```python
from build123d import *

# Parameters (mm, degrees)
SKETCH1_R           = 101.6
BOSS_EXTRUDE1_DEPTH = 457.2
SKETCH2_W           = 3.175
SKETCH2_H           = 88.9
BOSS_EXTRUDE3_DEPTH = 139.7
SKETCH2_3_W         = 88.9
SKETCH2_3_H         = 88.9
BOSS_EXTRUDE4_DEPTH = 3.175


with BuildPart() as part:
    # Sketch1 → Boss-Extrude1 (new body)
    with BuildSketch(Plane(origin=(0, 0, 0), x_dir=(1, 0, 0), z_dir=(0, 1, 0))):
        Circle(SKETCH1_R)
    extrude(amount=BOSS_EXTRUDE1_DEPTH)

    # Sketch2 → Boss-Extrude3 (add)
    with BuildSketch(Plane(origin=(0, 457.2, 0), x_dir=(1, 0, 0), z_dir=(0, 1, 0))):
        with Locations((46.0375, 0)):
            Rectangle(SKETCH2_W, SKETCH2_H)
        with Locations((-46.0375, 0)):
            Rectangle(SKETCH2_W, SKETCH2_H)
    extrude(amount=BOSS_EXTRUDE3_DEPTH)

    # Sketch2<3> → Boss-Extrude4 (add)
    with BuildSketch(Plane(origin=(0, 457.2, 0), x_dir=(1, 0, 0), z_dir=(0, 1, 0))):
        Rectangle(SKETCH2_3_W, SKETCH2_3_H)
    extrude(amount=BOSS_EXTRUDE4_DEPTH)


solid = part.part
```
Model file for the job. Use its own axes, mm. A direction names the side the tool comes from. Coordinates: 2 decimals unless noted, no trailing zeros. Order: outer loops, then holes, each group sorted by start corner. A loop starts at its lowest first (then second) coordinate and runs counter-clockwise, first axis right, second up. Notation, with made-up numbers: (-20, 60) -> (-8, 60) arc R23 cw to (-8, 89) -> close; hole circle Ø9 at (57.5, 80). An arc over 180 degrees is marked (long way). Answer as a JSON object with one key per item and string values. Group by question number.
1) Cut at D-D, the plane y = 219. Write the cut outline in (x, z).
2) Pull direction X, two halves, no side cores. Call faces 1 (the face through (-1, 457.2, -47)), 2 (the face through (-47.625, 526, 1)), 3 (the face through (-1, 460.375, -1)): +X half, -X half, draft (parallel to the pull), parting line (faces both ways), or undercut.
3) Cut at B-B, the plane x = 0. Write the cut outline in (y, z) (3 decimals).
4) Cut at A-A, the plane y = 469.5. Write the cut outline in (x, z) (3 decimals), then the cut area to 3 significant figures.
5) Cut at C-C, the plane z = 0. Write the cut outline in (x, y) (3 decimals), then the cut area to 3 significant figures.
6) Flat gauge pins, fed straight in: pin 1 (1.5 mm diameter, centred on y = 426, z = 6.5, fed in from +X); pin 2 (6 mm diameter, centred on x = 50, z = 51.5, fed in from +Y); pin 3 (10 mm diameter, centred on y = 472.5, z = -10.5, fed in from +X) (3 decimals); pin 4 (10 mm diameter, centred on x = 63, z = -74, fed in from -Y). Where does each tip first touch, or does it go through?
7) Drill centre lines: L1, parallel to X at y = 543.5, z = 30 (3 decimals); L2, parallel to Y at x = 40, z = 62; L3, parallel to Y at x = 1, z = -31 (3 decimals). Where is each one in solid material? Low to high.
8) Which spindle directions (+Z, -Z, +X, -X, +Y, -Y) get a long thin tool onto all of the face, cutting with end or side? Do faces 4 (the face through (-46, 506, -44.45)), 5 (the face through (46, 506, 44.45)), 6 (the face through (-22.025, 225.4, 99.184)), 7 (the face through (47.625, 526, 1)), 8 (the face through (-44.45, 528, 1)). Say none if no direction does.
Check values:
{
 "1": {"outline": "circle Ø203.2 at (0, 0)"},
 "2": {"face 1": "draft", "face 2": "-X half", "face 3": "undercut"},
 "3": {"outline": "(0, -101.6) -> (457.2, -101.6) -> (457.2, -44.45) -> (460.375, -44.45) -> (460.375, 44.45) -> (457.2, 44.45) -> (457.2, 101.6) -> (0, 101.6) -> close"},
 "4": {"outline": "(-47.625, -44.45) -> (-44.45, -44.45) -> (-44.45, 44.45) -> (-47.625, 44.45) -> close; (44.45, -44.45) -> (47.625, -44.45) -> (47.625, 44.45) -> (44.45, 44.45) -> close", "area": "565 mm²"},
 "5": {"outline": "(-101.6, 0) -> (101.6, 0) -> (101.6, 457.2) -> (47.625, 457.2) -> (47.625, 596.9) -> (44.45, 596.9) -> (44.45, 460.375) -> (-44.45, 460.375) -> (-44.45, 596.9) -> (-47.625, 596.9) -> (-47.625, 457.2) -> (-101.6, 457.2) -> close", "area": "94,100 mm²"},
 "6": {"pin 1": "stops at x = 101.44", "pin 2": "stops at y = 457.2", "pin 3": "stops at x = 47.625", "pin 4": "stops at y = 0"},
 "7": {"L1": "x = -47.625 to -44.45, 44.45 to 47.625", "L2": "y = 0 to 457.2", "L3": "y = 0 to 460.375"},
 "8": {"face 4": "-Z, +X, -X, +Y", "face 5": "+Z, +X, -X, +Y", "face 6": "+Y, -Y", "face 7": "+Z, -Z, +X, +Y", "face 8": "+Z, -Z, +Y"}
}
